from build123d import *

# Parameters (mm, degrees)
F3_DEPTH = 2
F4_DEPTH = 2
F5_DEPTH = 2


with BuildPart() as f3:
    # F1 (on Right) → F3 (new body)
    with BuildSketch(Plane.YZ):
        Polygon((-30, 0), (10, 0), (10, 50), (0, 50), (0, 40), (-30, 10), align=None)
    extrude(amount=F3_DEPTH)

    # F0 (on Top) → F4 (join)
    with BuildSketch(Plane.XY):
        Polygon((0, 10), (0, -30), (10, -30), (40, 0), (50, 0), (50, 10), align=None)
    extrude(amount=F4_DEPTH)

    # F2 (on Front) → F5 (join)
    with BuildSketch(Plane.XZ):
        Polygon((0, 0), (40, 0), (50, 0), (50, 10), (10, 10), (10, 50), (0, 50), (0, 40), align=None)
    extrude(amount=-F5_DEPTH)


solid = f3.part
Input: part model. Units: mm. Frame: model coordinates. A direction names the side the tool comes from. Coordinates: 2 decimals unless noted, no trailing zeros. Loops run counter-clockwise (first coordinate to the right, second up) from the corner with the lowest first, then second, coordinate; pieces in that order, holes last.
Q1. Material intervals for line 1 (Z direction, x = 23, y = -15.5), sorted ascending.
Q2. Cut plane A-A (x = 21). Output: boundary loops of the cut face in (y, z), then the cut area to 3 significant figures.
Q3. Cut plane D-D (x = 43.5). Output: boundary loops of the cut face in (y, z).
Q4. Set-up query: faces 1 (the face through (14, 0, 8)), 2 (the face through (30, 1, 10)), 3 (the face through (8, 2, 17)), 4 (the face through (0, -6, 20)). Return all of +Z, -Z, +X, -X, +Y, -Y with unobstructed straight access to the full face (end or side cutting, diameter ignored); none if empty.
Q5. Contact query for flat-ended pins moving along their axis: pin 1 (3 mm diameter, centred on x = 8, z = 17.5, fed in from +Y); pin 2 (4 mm diameter, centred on y = -13, z = 15, fed in from +X); pin 3 (6.5 mm diameter, centred on x = 28.5, y = 8, fed in from +Z). Output: stop coordinate, or through.
Q6. Cut plane C-C (y = 4). Output: boundary loops of the cut face in (x, z).
Q7. Cut plane B-B (z = 34). Output: boundary loops of the cut face in (x, y).
Working result:
1. line 1: z = 0 to 2
2. outline: (-19, 0) - (10, 0) - (10, 2) - (2, 2) - (2, 10) - (0, 10) - (0, 2) - (-19, 2) - close
2. area: 74.0 mm2
3. outline: (0, 0) - (10, 0) - (10, 2) - (2, 2) - (2, 10) - (0, 10) - close
4. face 1: +Z, +X, -Y
4. face 2: +Z, +X, +Y, -Y
4. face 3: +Z, +X, +Y
4. face 4: +Z, -Z, -X, +Y, -Y
5. pin 1: stops at y = 2
5. pin 2: stops at x = 2
5. pin 3: stops at z = 2
6. outline: (0, 0) - (50, 0) - (50, 2) - (2, 2) - (2, 50) - (0, 50) - close
7. outline: (0, -6) - (2, -6) - (2, 0) - (10, 0) - (10, 2) - (2, 2) - (2, 10) - (0, 10) - close
